Source: CAD feature listing. Evaluate the final solid. Frame: model axes, mm. Give positions to 0.01 mm unless a question says otherwise; leave off trailing zeros. Write each loop counter-clockwise with the first axis right and the second up, starting at its lowest first coordinate (ties: lowest second). Pieces come first, ordered by that corner, then holes. Notation, with made-up numbers: (-26.75, -1.75) - (27.25, -1.75) arc R28 cw to (27.25, 20.25) - close; hole circle Ø1 at (48, 59.25). An arc over 180 degrees is marked (long way). Answer as a JSON object with one key per item and string values. Group by question number.
from build123d import *

# Parameters (mm, degrees)
ESBO_O1_W                = 28
ESBO_O1_H                = 15
ESBO_O1_R                = 1.5
RESSALTO_EXTRUS_O1_DEPTH = 15
FILETE1_R                = 5


with BuildPart() as part:
    # Esboço1 → Ressalto-extrusão1 (new body)
    with BuildSketch(Plane.XY):
        Rectangle(ESBO_O1_W, ESBO_O1_H)
        with Locations((-8, 0)):
            Circle(ESBO_O1_R, mode=Mode.SUBTRACT)
        with Locations((8, 0)):
            Circle(ESBO_O1_R, mode=Mode.SUBTRACT)
    extrude(amount=RESSALTO_EXTRUS_O1_DEPTH)

    # Filete1
    filete1_edges = [part.edges().sort_by_distance(p)[0] for p in [
        (14, -7.5, 7.5),
        (-14, -7.5, 7.5),
        (-14, 7.5, 7.5),
        (14, 7.5, 7.5),
    ]]
    fillet(filete1_edges, radius=FILETE1_R)


solid = part.part
Q1. Section B-B on x = 8. Return the cut outline in (y, z).
Q2. Section C-C on z = 11.25. Return the cut outline in (x, y).
Q3. Draft query along Y for faces 1 (the flat face through (14, 0, 7)), 2 (the cylindrical face through (6.5, 0.07, 7.4)), 3 (the cylindrical face through (12.5, -6.07, 7.6)). Return one class per face: released by +Y, released by -Y, zero draft, split by the parting line, or undercut.
Q4. Section A-A on y = 0. Return the cut outline in (x, z).
Q5. Section D-D on y = 6.5. Return the cut outline in (x, z).
Q6. Ray query, probe 1 along Y at (x, z) = (-8, 9.75); probe 2 along X at (y, z) = (-0.25, 1); probe 3 along X at (y, z) = (1, 7). Return the intervals inside material, ascending. Write a range as [from, to].
Taken from the geometry:
{
 "1": {"outline": "(-7.5, 0) - (-1.5, 0) - (-1.5, 15) - (-7.5, 15) - close; (1.5, 0) - (7.5, 0) - (7.5, 15) - (1.5, 15) - close"},
 "2": {"outline": "(-14, -2.5) arc R5 ccw to (-9, -7.5) - (9, -7.5) arc R5 ccw to (14, -2.5) - (14, 2.5) arc R5 ccw to (9, 7.5) - (-9, 7.5) arc R5 ccw to (-14, 2.5) - close; hole circle Ø3 at (-8, 0); hole circle Ø3 at (8, 0)"},
 "3": {"face 1": "zero draft", "face 2": "undercut", "face 3": "released by -Y"},
 "4": {"outline": "(-14, 0) - (-9.5, 0) - (-9.5, 15) - (-14, 15) - close; (-6.5, 0) - (6.5, 0) - (6.5, 15) - (-6.5, 15) - close; (9.5, 0) - (14, 0) - (14, 15) - (9.5, 15) - close"},
 "5": {"outline": "(-12, 0) - (12, 0) - (12, 15) - (-12, 15) - close"},
 "6": {"probe 1": "y = [-7.5, -1.5], [1.5, 7.5]", "probe 2": "x = [-14, -9.48], [-6.52, 6.52], [9.48, 14]", "probe 3": "x = [-14, -9.12], [-6.88, 6.88], [9.12, 14]"}
}
